Part model, mm, in its own coordinate system. A direction names the side the tool comes from. Round coordinates to 2 decimals unless told otherwise and drop trailing zeros. Order: outer loops, then holes, each group sorted by start corner. A loop starts at its lowest first (then second) coordinate and runs counter-clockwise, first axis right, second up. Notation, with made-up numbers: (8.5, 55) -> (13.5, 55) arc R20 ccw to (13.5, 68) -> close; hole circle Ø4 at (37, 24). An arc over 180 degrees is marked (long way). Answer as a JSON object with one key per item and string values. Group by question number.
```python
from build123d import *

# Parameters (mm, degrees)
BOSS_EXTRUDE1_START = -4.5
SKETCH1_R           = 0.8
BOSS_EXTRUDE1_DEPTH = 7.5
FILLET1_R           = 4
SKETCH4_W           = 10.5
SKETCH4_H           = 4.5
CUT_EXTRUDE2_DEPTH  = 29.619267985
SKETCH5_W           = 15
SKETCH5_H           = 4.5
CUT_EXTRUDE3_DEPTH  = 29.619267985
FILLET2_R           = 10
FILLET3_R           = 5
FILLET4_R           = 5
SKETCH7_W           = 29.25
SKETCH7_H           = 14.263139721
CUT_EXTRUDE4_DEPTH  = 7.5
CUT_EXTRUDE5_START  = -6.755354819
CUT_EXTRUDE5_DEPTH  = 8.755354819
SKETCH10_R          = 1.51
CUT_EXTRUDE6_DEPTH  = 1.5


# Read off the part's stored shape, not the designer's step: Mirror5, Cut-Extrude5
with BuildPart() as part:
    # Sketch1 → Boss-Extrude1 (new body)
    with BuildSketch(Plane.XY.offset(BOSS_EXTRUDE1_START)):
        with BuildLine():
            Line((-4.389678411, -3.5), (-19.133343362, 6.422379894))
            ThreePointArc((-19.133343362, 6.422379894), (-19.666253628, 6.676053774), (-20.25, 6.763139721))
            Line((-20.25, 6.763139721), (-25.25, 6.763139721))
            ThreePointArc((-25.25, 6.763139721), (-27.246991207, 4.872803379), (-25.468997361, 2.775165839))
            ThreePointArc((-25.468997361, 2.775165839), (-25.359663658, 2.766148514), (-25.25, 2.763139721))
            Line((-25.25, 2.763139721), (-20.860321589, 2.763139721))
            Line((-20.860321589, 2.763139721), (-6.116656638, -7.159240173))
            ThreePointArc((-6.116656638, -7.159240173), (-5.583746372, -7.412914053), (-5, -7.5))
            Line((-5, -7.5), (0, -7.5))
            ThreePointArc((0, -7.5), (1.974370247, -5.81915847), (0.630136986, -3.601862129))
            ThreePointArc((0.630136986, -3.601862129), (0.31915847, -3.525629753), (0, -3.5))
            Line((0, -3.5), (-4.389678411, -3.5))
        make_face()
        with Locations((0, -5.5)):
            Circle(SKETCH1_R, mode=Mode.SUBTRACT)
        with Locations((-25.25, 4.763139721)):
            Circle(SKETCH1_R, mode=Mode.SUBTRACT)
    extrude(amount=BOSS_EXTRUDE1_DEPTH)

    # Fillet1
    fillet1_edges = [part.edges().sort_by_distance(p)[0] for p in [
        (-4.389678411, -3.5, -0.75),
        (-20.860321589, 2.763139721, -0.75),
    ]]
    fillet(fillet1_edges, radius=FILLET1_R)

    # Sketch4 → Cut-Extrude2 (cut, symmetric)
    with BuildSketch(Plane(origin=(0, 0, 0), x_dir=(1, 0, 0), z_dir=(0, 1, 0))):
        with Locations((-3.25, 2.25)):
            Rectangle(SKETCH4_W, SKETCH4_H)
    extrude(amount=CUT_EXTRUDE2_DEPTH, both=True, mode=Mode.SUBTRACT)

    # Sketch5 → Cut-Extrude3 (cut, symmetric)
    with BuildSketch(Plane(origin=(0, 0, 0), x_dir=(1, 0, 0), z_dir=(0, 1, 0))):
        with Locations((-19.75, -0.75)):
            Rectangle(SKETCH5_W, SKETCH5_H)
    extrude(amount=CUT_EXTRUDE3_DEPTH, both=True, mode=Mode.SUBTRACT)

    # Fillet2
    # the kernel refuses this fillet: 10 mm, written as the material it takes off along each edge
    with BuildSketch(Plane(origin=(-12.25, -23.910660804, 3), x_dir=(1.537930276954748e-12, 0, -1.0), z_dir=(0, 1, 0))) as fillet2_piece_1:
        with BuildLine():
            CenterArc((10, -8.351646544), FILLET2_R, 123.367012969, 56.632987031)
            Line((0, -8.351646544), (-0.2, -8.351646544))
            Line((-0.2, -8.351646544), (-0.2, 0))
            Line((-0.2, 0), (0, 0.2))
            ThreePointArc((0, 0.2), (2.25, 0.2), (4.39, 0.167032931))
            Line((4.39, 0.167032931), (4.5, 0))
        make_face()
    extrude(amount=46.579716753, mode=Mode.SUBTRACT)

    # Fillet3
    # the kernel refuses this fillet: 5 mm, written as the material it takes off along each edge
    with BuildSketch(Plane(origin=(-8.5, -17.99261029, -4.5), x_dir=(0, 0, 1), z_dir=(0, 1, 0))) as fillet3_piece_1:
        with BuildLine():
            CenterArc((5, -4.974937186), FILLET3_R, 95.739170477, 84.260829523)
            Line((0, -4.974937186), (-0.1, -4.974937186))
            Line((-0.1, -4.974937186), (-0.1, 0))
            Line((-0.1, 0), (0, 0.1))
            ThreePointArc((0, 0.1), (2.25, 0.1), (4.49, 0.099498744))
            Line((4.49, 0.099498744), (4.5, 0))
        make_face()
    extrude(amount=29.696169959, mode=Mode.SUBTRACT)

    # Fillet4
    fillet4_edges = [part.edges().sort_by_distance(p)[0] for p in [
        (-12.25, -0.620802428, -1.5),
    ]]
    fillet(fillet4_edges, radius=FILLET4_R)

    # Mirror5: part across plane


with BuildPart() as part_1:
    add(part.part)
    add(part.part.mirror(Plane.XY.offset(-4.5)))

    # Sketch7 → Cut-Extrude4 (cut)
    with BuildSketch(Plane.XY.offset(3)):
        with Locations((-12.625, -0.36843014)):
            Rectangle(SKETCH7_W, SKETCH7_H)
    extrude(amount=-CUT_EXTRUDE4_DEPTH, mode=Mode.SUBTRACT)

    # Cut-Extrude5 outline → Cut-Extrude5 (cut)
    with BuildSketch(Plane(origin=(0, 0, 0), x_dir=(0, 0, -1), z_dir=(1, 0, 0)).offset(CUT_EXTRUDE5_START)):
        with BuildLine():
            add(Edge.make_bspline(
                [(10.5, -7.5), (12, -7.5), (12, -5)],
                knots=[0, 0, 0, 1.570796327, 1.570796327, 1.570796327], degree=2, weights=[1, 0.707106781, 1]))
            Line((10.5, -7.5), (12, -7.5))
            Line((12, -7.5), (12, -5))
        make_face()
    extrude(amount=CUT_EXTRUDE5_DEPTH, mode=Mode.SUBTRACT)

    # Sketch10 → Cut-Extrude6 (cut)
    with BuildSketch(Plane(origin=(0, 0, -12), x_dir=(-1, 0, 0), z_dir=(0, 0, -1))):
        with Locations((0, -5.5)):
            Circle(SKETCH10_R)
    extrude(amount=-CUT_EXTRUDE6_DEPTH, mode=Mode.SUBTRACT)


solid = part_1.part
```
Q1. Wall check: line 1 (Y direction, x = -25.25, z = -6.2); line 2 (Z direction, x = -15.5, y = -0.5); line 3 (X direction, y = -5.5, z = -11.2). Give the ranges that are in metal, low to high. Write a range as [from, to].
Q2. Band-saw the part on D-D (x = -16.75). List the corners of the cut face in (y, z), plus the area to 3 significant figures.
Q3. Band-saw the part on B-B (x = -12). List the corners of the cut face in (y, z), plus the area to 3 significant figures.
Q4. Band-saw the part on C-C (z = -10). List the corners of the cut face in (x, y).
Q5. Band-saw the part on A-A (z = -6). List the corners of the cut face in (x, y), plus the area to 3 significant figures.
Q6. Drop flat-ended pins along their axis: pin 1 Ø0.9 at (x, y) = (0, -5) entering from -Z; pin 2 Ø2 at (x, y) = (-24, 0.5) entering from -Z; pin 3 Ø6.5 at (x, y) = (-23.5, 1.5) entering from -Z; pin 4 Ø0.9 at (x, z) = (-23, -5.5) entering from -Y. Give the stop position or say it passes through.
Q7. Which spindle directions (+Z, -Z, +X, -X, +Y, -Y) get a long thin tool onto all of the face, cutting with end or side? Do faces 4 (the cylindrical face through (0.197, -4.003, -11.26)), 5 (the flat face through (-24, 2.763, -6)), 6 (the flat face through (-20, 4, -7.5)), 7 (the flat face through (-3, -5, -9)), 8 (the cylindrical face through (-4.35, -3.32, -10.52)). Say none if no direction does.
Q8. Two-plate mould, pull along Y, no slides. Class faces 1 (the cylindrical face through (-19.658, 6.674, -5.979)), 2 (the cylindrical face through (-0.17, -6.28, -9.74)), 3 (the flat face through (-3, -7.5, -10)): +Y half, -Y half, draft (parallel to the pull), parting line (faces both ways), or undercut.
Completed:
{
 "1": {"line 1": "[2.76, 3.96], [5.56, 6.76]", "line 2": "[-7.5, -4.5]", "line 3": "[-7.82, -1.51], [1.51, 2]"},
 "2": {"outline": "(0, -7.5) -> (4.82, -7.5) -> (4.82, -4.5) -> (0, -4.5) -> close", "area": "14.5 mm2"},
 "3": {"outline": "(-3.2, -8.24) -> (1.62, -8.24) -> (1.62, -4.72) -> (-3.2, -4.72) -> close", "area": "16.9 mm2"},
 "4": {"outline": "(-9.9, -4.61) -> (-6.12, -7.16) arc R2 ccw to (-5, -7.5) -> (0, -7.5) arc R2 ccw to (0, -3.5) -> (-3.17, -3.5) arc R4 cw to (-5.4, -2.82) -> (-9.9, 0.21) -> close; hole circle Ø1.6 at (0, -5.5)"},
 "5": {"outline": "(-25.25, 2.76) -> (-22.08, 2.76) arc R4 cw to (-19.85, 2.08) -> (-9.9, -4.61) -> (-9.9, 0.21) -> (-19.13, 6.42) arc R2 ccw to (-20.25, 6.76) -> (-25.25, 6.76) arc R2 ccw to start; hole circle Ø1.6 at (-25.25, 4.76)", "area": "74.3 mm2"},
 "6": {"pin 1": "z = -10.5", "pin 2": "through", "pin 3": "z = -7.5", "pin 4": "y = 2.76"},
 "7": {"face 4": "-Z", "face 5": "+Z, -Z, -X, -Y", "face 6": "-Z, -X, +Y, -Y", "face 7": "+Z, +X, +Y, -Y", "face 8": "+Z, -Z, +X, +Y"},
 "8": {"face 1": "+Y half", "face 2": "undercut", "face 3": "-Y half"}
}
